Source: CAD feature listing. Evaluate the final solid. Frame: model axes, mm. Coordinates: 2 decimals unless noted, no trailing zeros. Order: outer loops, then holes, each group sorted by start corner. A loop starts at its lowest first (then second) coordinate and runs counter-clockwise, first axis right, second up.
Item 1: Ray query, line 1 (X direction, y = -0.3, z = 5); line 2 (X direction, y = 0.3, z = -32.26); line 3 (Z direction, x = -5.5, y = 0.2). Return the intervals inside material, ascending.
Item 2: Section C-C on y = -0.5. State how many separate pieces and enclosed holes the cut face has, then the cut area to 3 significant figures.
Item 3: Contact query for flat-ended pins moving along their axis: P1, Ø0.5, axis at y = 0.5, z = -44, coming from the -X side; P2, Ø0.8, axis at x = -38, y = 0, coming from the -Z side; P3, Ø0.8, axis at x = 48.5, y = 0, coming from the -Z side. Output: stop coordinate, or through.
Item 4: Section B-B on z = -5. Return the cut outline in (x, y), then the cut area to 3 significant figures.
Item 5: Section A-A on x = -32.26. Return the cut outline in (y, z).
Item 6: Mould query, pull axis X, two halves, no side actions, for faces 1 (the flat face through (-1, -0.8, -3)), 2 (the cylindrical face through (31.1, 0, 4.7)), 3 (the flat face through (-47, 0, 41.9)). Classes: released by +X, released by -X, zero draft, split by the parting line, or undercut.
from build123d import *

# Parameters (mm, degrees)
GENERICCARDPCBDEFINITION_START = -0.8
GENERICCARDPCBDEFINITION_DEPTH = 1.6
CUT_EXTRUDE1_REACH             = 72.587
SKETCH1_R                      = 1.2


# Read off the part's stored shape, not the designer's step: GenericCardPCBDefinition
with BuildPart() as part:
    # GenericCardPCBDefinition outline → GenericCardPCBDefinition (new body)
    with BuildSketch(Plane(origin=(0, 0, 0), x_dir=(1, 0, 0), z_dir=(0, 1, 0)).offset(GENERICCARDPCBDEFINITION_START)):
        with BuildLine():
            Line((-49.9, -39), (-44.1, -44.8))
            Line((-44.1, -44.8), (-41.232050808, -44.8))
            ThreePointArc((-41.232050808, -44.8), (-39.5, -43.8), (-37.767949192, -44.8))
            Line((-37.767949192, -44.8), (-18.232050808, -44.8))
            ThreePointArc((-18.232050808, -44.8), (-16.5, -43.8), (-14.767949192, -44.8))
            Line((-14.767949192, -44.8), (14.767949192, -44.8))
            ThreePointArc((14.767949192, -44.8), (16.5, -43.8), (18.232050808, -44.8))
            Line((18.232050808, -44.8), (37.767949192, -44.8))
            ThreePointArc((37.767949192, -44.8), (39.5, -43.8), (41.232050808, -44.8))
            Line((41.232050808, -44.8), (44.1, -44.8))
            Line((44.1, -44.8), (49.9, -39))
            Line((49.9, -39), (49.9, 40.7))
            ThreePointArc((49.9, 40.7), (49.753553391, 41.053553391), (49.4, 41.2))
            Line((49.4, 41.2), (47.65, 41.2))
            ThreePointArc((47.65, 41.2), (47.296446609, 41.346446609), (47.15, 41.7))
            Line((47.15, 41.7), (47.15, 45.8))
            ThreePointArc((47.15, 45.8), (47.003553391, 46.153553391), (46.65, 46.3))
            Line((46.65, 46.3), (34.9, 46.3))
            ThreePointArc((34.9, 46.3), (34.546446609, 46.446446609), (34.4, 46.8))
            Line((34.4, 46.8), (34.4, 49.4))
            ThreePointArc((34.4, 49.4), (34.253553391, 49.753553391), (33.9, 49.9))
            Line((33.9, 49.9), (-33.9, 49.9))
            ThreePointArc((-33.9, 49.9), (-34.253553391, 49.753553391), (-34.4, 49.4))
            Line((-34.4, 49.4), (-34.4, 46.8))
            ThreePointArc((-34.4, 46.8), (-34.546446609, 46.446446609), (-34.9, 46.3))
            Line((-34.9, 46.3), (-46.65, 46.3))
            ThreePointArc((-46.65, 46.3), (-47.003553391, 46.153553391), (-47.15, 45.8))
            Line((-47.15, 45.8), (-47.15, 41.7))
            ThreePointArc((-47.15, 41.7), (-47.296446609, 41.346446609), (-47.65, 41.2))
            Line((-47.65, 41.2), (-49.4, 41.2))
            ThreePointArc((-49.4, 41.2), (-49.753553391, 41.053553391), (-49.9, 40.7))
            Line((-49.9, 40.7), (-49.9, -39))
        make_face()
    extrude(amount=GENERICCARDPCBDEFINITION_DEPTH)

    # Sketch1 → Cut-Extrude1 (cut, up to next)
    with BuildSketch(Plane(origin=(0, 0.8, 0), x_dir=(1, 0, 0), z_dir=(0, 1, 0)), mode=Mode.PRIVATE) as cut_extrude1_sk1:
        with Locations(Location((32.26, 5, 0), (0, 0, 270))):
            Circle(SKETCH1_R)
    cut_extrude1_tool1 = extrude(cut_extrude1_sk1.sketch, amount=-CUT_EXTRUDE1_REACH, mode=Mode.PRIVATE) & part.part
    # Sketch1 → Cut-Extrude1 (cut, up to next)
    with BuildSketch(Plane(origin=(0, 0.8, 0), x_dir=(1, 0, 0), z_dir=(0, 1, 0)), mode=Mode.PRIVATE) as cut_extrude1_sk2:
        with Locations(Location((32.26, -5, 0), (0, 0, 270))):
            Circle(SKETCH1_R)
    cut_extrude1_tool2 = extrude(cut_extrude1_sk2.sketch, amount=-CUT_EXTRUDE1_REACH, mode=Mode.PRIVATE) & part.part
    # Sketch1 → Cut-Extrude1 (cut, up to next)
    with BuildSketch(Plane(origin=(0, 0.8, 0), x_dir=(1, 0, 0), z_dir=(0, 1, 0)), mode=Mode.PRIVATE) as cut_extrude1_sk3:
        with Locations(Location((-32.26, 5, 0), (0, 0, 270))):
            Circle(SKETCH1_R)
    cut_extrude1_tool3 = extrude(cut_extrude1_sk3.sketch, amount=-CUT_EXTRUDE1_REACH, mode=Mode.PRIVATE) & part.part
    # Sketch1 → Cut-Extrude1 (cut, up to next)
    with BuildSketch(Plane(origin=(0, 0.8, 0), x_dir=(1, 0, 0), z_dir=(0, 1, 0)), mode=Mode.PRIVATE) as cut_extrude1_sk4:
        with Locations(Location((-32.26, -5, 0), (0, 0, 270))):
            Circle(SKETCH1_R)
    cut_extrude1_tool4 = extrude(cut_extrude1_sk4.sketch, amount=-CUT_EXTRUDE1_REACH, mode=Mode.PRIVATE) & part.part
    # Sketch1 → Cut-Extrude1 (cut, up to next)
    with BuildSketch(Plane(origin=(0, 0.8, 0), x_dir=(1, 0, 0), z_dir=(0, 1, 0)), mode=Mode.PRIVATE) as cut_extrude1_sk5:
        with Locations(Location((-5, -32.26, 0), (0, 0, 270))):
            Circle(SKETCH1_R)
    cut_extrude1_tool5 = extrude(cut_extrude1_sk5.sketch, amount=-CUT_EXTRUDE1_REACH, mode=Mode.PRIVATE) & part.part
    # Sketch1 → Cut-Extrude1 (cut, up to next)
    with BuildSketch(Plane(origin=(0, 0.8, 0), x_dir=(1, 0, 0), z_dir=(0, 1, 0)), mode=Mode.PRIVATE) as cut_extrude1_sk6:
        with Locations(Location((5, -32.26, 0), (0, 0, 270))):
            Circle(SKETCH1_R)
    cut_extrude1_tool6 = extrude(cut_extrude1_sk6.sketch, amount=-CUT_EXTRUDE1_REACH, mode=Mode.PRIVATE) & part.part
    # Sketch1 → Cut-Extrude1 (cut, up to next)
    with BuildSketch(Plane(origin=(0, 0.8, 0), x_dir=(1, 0, 0), z_dir=(0, 1, 0)), mode=Mode.PRIVATE) as cut_extrude1_sk7:
        with Locations(Location((-5, 32.26, 0), (0, 0, 270))):
            Circle(SKETCH1_R)
    cut_extrude1_tool7 = extrude(cut_extrude1_sk7.sketch, amount=-CUT_EXTRUDE1_REACH, mode=Mode.PRIVATE) & part.part
    # Sketch1 → Cut-Extrude1 (cut, up to next)
    with BuildSketch(Plane(origin=(0, 0.8, 0), x_dir=(1, 0, 0), z_dir=(0, 1, 0)), mode=Mode.PRIVATE) as cut_extrude1_sk8:
        with Locations(Location((5, 32.26, 0), (0, 0, 270))):
            Circle(SKETCH1_R)
    cut_extrude1_tool8 = extrude(cut_extrude1_sk8.sketch, amount=-CUT_EXTRUDE1_REACH, mode=Mode.PRIVATE) & part.part
    add(cut_extrude1_tool1.solids().sort_by_distance((32.26, 0.8, -5))[0], mode=Mode.SUBTRACT)
    add(cut_extrude1_tool2.solids().sort_by_distance((32.26, 0.8, 5))[0], mode=Mode.SUBTRACT)
    add(cut_extrude1_tool3.solids().sort_by_distance((-32.26, 0.8, -5))[0], mode=Mode.SUBTRACT)
    add(cut_extrude1_tool4.solids().sort_by_distance((-32.26, 0.8, 5))[0], mode=Mode.SUBTRACT)
    add(cut_extrude1_tool5.solids().sort_by_distance((-5, 0.8, 32.26))[0], mode=Mode.SUBTRACT)
    add(cut_extrude1_tool6.solids().sort_by_distance((5, 0.8, 32.26))[0], mode=Mode.SUBTRACT)
    add(cut_extrude1_tool7.solids().sort_by_distance((-5, 0.8, -32.26))[0], mode=Mode.SUBTRACT)
    add(cut_extrude1_tool8.solids().sort_by_distance((5, 0.8, -32.26))[0], mode=Mode.SUBTRACT)


solid = part.part
Answer list:
1. line 1: x = -49.9 to -33.46, -31.06 to 31.06, 33.46 to 49.9
1. line 2: x = -49.9 to -6.2, -3.8 to 3.8, 6.2 to 49.9
1. line 3: z = -49.9 to -33.35, -31.17 to 31.17, 33.35 to 44.8
2. separate pieces: 1
2. enclosed holes: 8
2. area: 9,230 mm2
3. P1: stops at x = -47.15
3. P2: stops at z = -46.3
3. P3: stops at z = -41.2
4. outline: (-49.9, -0.8) - (-33.46, -0.8) - (-33.46, 0.8) - (-49.9, 0.8) - close; (-31.06, -0.8) - (31.06, -0.8) - (31.06, 0.8) - (-31.06, 0.8) - close; (33.46, -0.8) - (49.9, -0.8) - (49.9, 0.8) - (33.46, 0.8) - close
4. area: 152 mm2
5. outline: (-0.8, -49.9) - (0.8, -49.9) - (0.8, -6.2) - (-0.8, -6.2) - close; (-0.8, -3.8) - (0.8, -3.8) - (0.8, 3.8) - (-0.8, 3.8) - close; (-0.8, 6.2) - (0.8, 6.2) - (0.8, 44.8) - (-0.8, 44.8) - close
6. face 1: zero draft
6. face 2: undercut
6. face 3: released by -X
